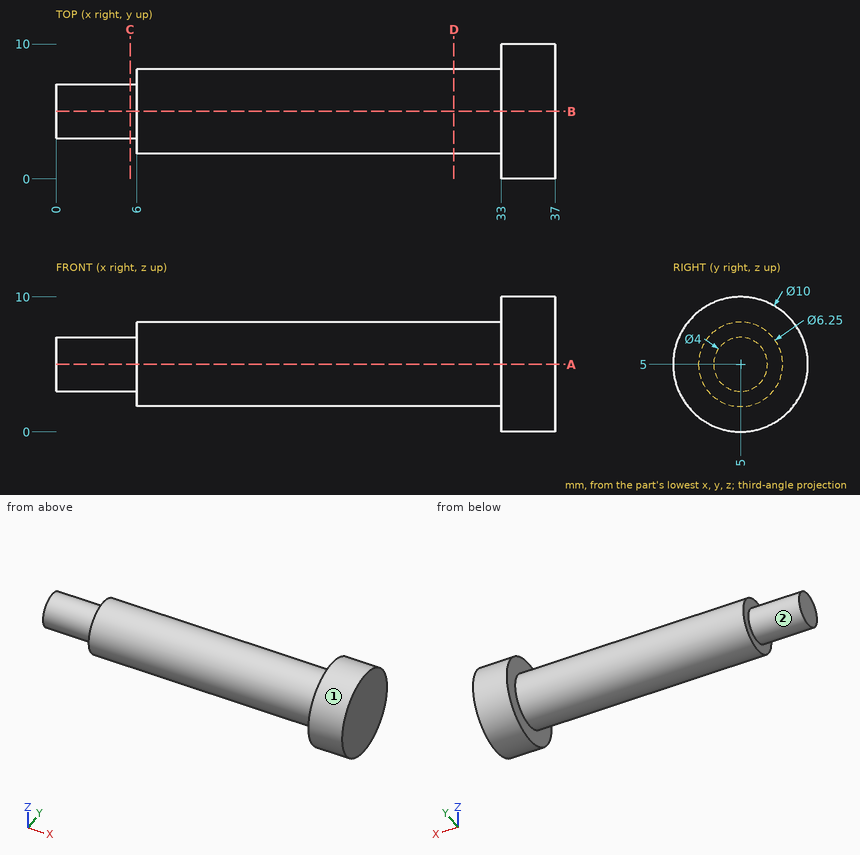
Answer from the drawing. Dimensions are ordinates in mm from the lowest x, y and z of the part. A direction names the side the tool comes from. Coordinates: 2 decimals unless noted, no trailing zeros. Order: outer loops, then holes, each group sorted by start corner. A loop starts at its lowest first (then second) coordinate and runs counter-clockwise, first axis right, second up. Notation, with made-up numbers: M 44,18.5 L 101,18.5 A10 cw 101,30.5 Z; hole C -10.5,68.5 d3. An arc over 180 degrees is marked long. Put each result on its own line as item: value. Start each with the question number.
Item 1: Section A-A, the plane z = 5 is taken. Determine the outline of the cut face in (x, y) (3 decimals), plus the area to 3 significant figures.
Item 2: Given pin 1 Ø4 at (x, y) = (5.5, 5.5) entering from +Z (3 decimals); pin 2 Ø1.5 at (x, z) = (8, 1.5) entering from +Y; pin 3 Ø6 at (x, z) = (25, 9) entering from -Y; pin 4 Ø1.9 at (y, z) = (5, 5) entering from -X, each flat-ended and moving along its own axis, determine where each tip first touches the part or whether it passes through.
Item 3: Section D-D, the plane x = 29.5 is taken. Determine the outline of the cut face in (y, z) (3 decimals), plus the area to 3 significant figures.
Item 4: For the marked faces 1 and 2, determine the directions among +Z, -Z, +X, -X, +Y, -Y from which every point of the face is accessible in a straight line to the end or side of a thin tool.
Item 5: Section C-C, the plane x = 5.5 is taken. Determine the outline of the cut face in (y, z), plus the area to 3 significant figures.
Item 6: Consider probe 1 along X at (y, z) = (5.5, 2); probe 2 along X at (y, z) = (2, 6.5); probe 3 along Z at (x, y) = (8, 6.5). Determine where each line is inside the solid, lowest interval first. Write a range as [from, to].
Computed:
1. outline: M 0,3 L 6,3 L 6,1.875 L 33,1.875 L 33,0 L 37,0 L 37,10 L 33,10 L 33,8.125 L 6,8.125 L 6,7 L 0,7 Z
1. area: 233 mm2
2. pin 1: stops at z = 8.125
2. pin 2: stops at y = 6.48
2. pin 3: stops at y = 2.04
2. pin 4: stops at x = 0
3. outline: C 5,5 d6.25
3. area: 30.7 mm2
4. face 1: +X, -X
4. face 2: -X
5. outline: C 5,5 d4
5. area: 12.6 mm2
6. probe 1: x = [6, 37]
6. probe 2: x = [33, 37]
6. probe 3: z = [2.26, 7.74]
